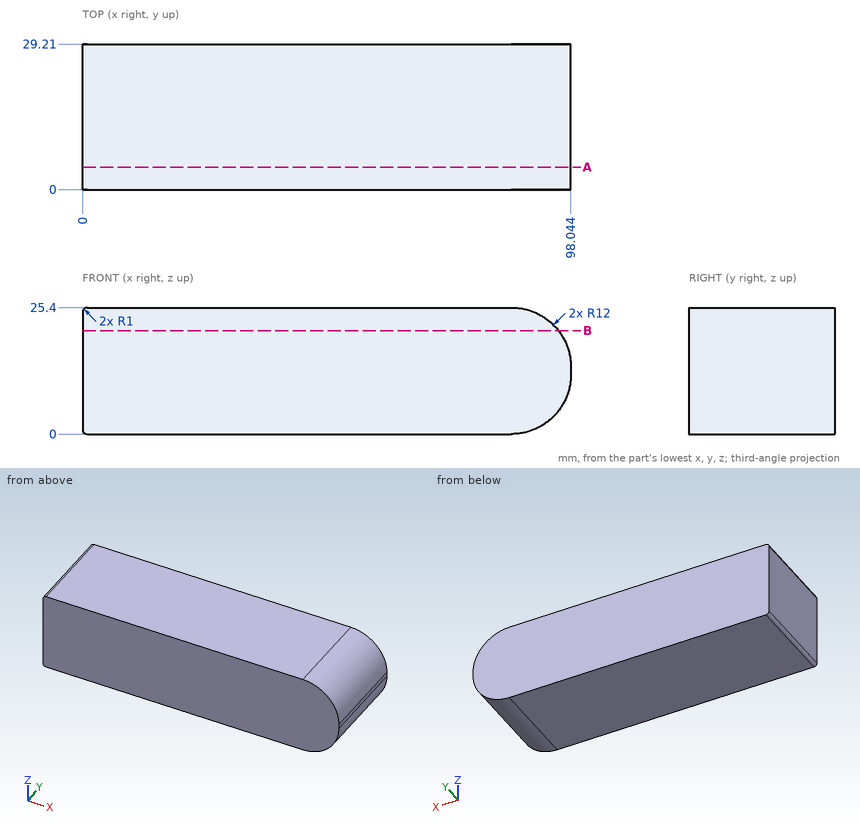
Input: dimensioned drawing with shaded views. Units: mm. Origin: part minimum x, y, z. Give positions to 0.01 mm unless a question says otherwise; leave off trailing zeros. Order: outer loops, then holes, each group sorted by start corner. A loop starts at its lowest first (then second) coordinate and runs counter-clockwise, first axis right, second up.
(1) Material intervals for line 1 along X through (y, z) = (7, 13.5); line 2 along X through (y, z) = (27, 21.5), sorted ascending.
(2) Section query A-A (y = 4.5). Return the cut outline in (x, z).
(3) Section query B-B (z = 20.75). Return the cut outline in (x, y), plus the area to 3 significant figures.
Outcome:
1. line 1: x = 0 to 98.04
1. line 2: x = 0 to 94.9
2. outline: (0, 1) arc R1 ccw to (1, 0) - (86.04, 0) arc R12 ccw to (98.04, 12) - (98.04, 13.4) arc R12 ccw to (86.04, 25.4) - (1, 25.4) arc R1 ccw to (0, 24.4) - close
3. outline: (0, 0) - (95.53, 0) - (95.53, 29.21) - (0, 29.21) - close
3. area: 2,790 mm2
